Source: CAD feature listing. Evaluate the final solid. Frame: model axes, mm. A direction names the side the tool comes from. Coordinates: 2 decimals unless noted, no trailing zeros. Order: outer loops, then holes, each group sorted by start corner. A loop starts at its lowest first (then second) coordinate and runs counter-clockwise, first axis right, second up.
Item 1: Ray query, line 1 (Y direction, x = 28, z = 20); line 2 (Y direction, x = 8, z = -8.5); line 3 (X direction, y = 14.5, z = 4). Return the intervals inside material, ascending.
Item 2: Contact query for flat-ended pins moving along their axis: P1, Ø5, axis at x = -14, y = 18.5, coming from the -Z side; P2, Ø12, axis at y = 11, z = 6.5, coming from the -X side; P3, Ø10, axis at x = 6, z = 3.5, coming from the +Y side; P4, Ø8, axis at x = -18, z = -24, coming from the -Y side. Output: stop coordinate, or through.
Item 3: Section C-C on y = 10. Return the cut outline in (x, z).
Item 4: Section D-D on x = 25.4. Return the cut outline in (y, z).
Item 5: Reachability of faces 1 (the flat face through (0, 12.7, 2)), 2 (the flat face through (0, -25.4, 0)) from +Z, -Z, +X, -X, +Y, -Y: full face, straight path, thin tool, end or side. Return the list, or none.
Item 6: Section A-A on x = 0. Return the cut outline in (y, z).
Item 7: Section B-B on z = 0. Return the cut outline in (x, y).
Item 8: Mould query, pull axis Z, two halves, no side actions, for faces 3 (the cylindrical face through (3.86, -12.52, -5.04)), 4 (the flat face through (0, 6, 14.665)), 5 (the flat face through (-12.61, 6.26, -7.49)), 6 (the flat face through (8, 0, 0)). Classes: released by +Z, released by -Z, zero draft, split by the parting line, or undercut.
from build123d import *

# Parameters (mm, degrees)
BOSS_EXTRUDE1_DEPTH = 12.7
SKETCH2_R           = 12.7
BOSS_EXTRUDE2_DEPTH = 12.7
SKETCH3_R           = 6.35
BOSS_EXTRUDE3_DEPTH = 25.4


with BuildPart() as part:
    # Sketch1 → Boss-Extrude1 (new body)
    with BuildSketch(Plane(origin=(0, 0, 0), x_dir=(1, 0, 0), z_dir=(0, 1, 0))):
        with BuildLine():
            Line((-6.35, 18.330871047), (-19.05, -3.666174209))
            ThreePointArc((-19.05, -3.666174209), (-36.398522628, -21.014696837), (-12.7, -14.664696837))
            Line((-12.7, -14.664696837), (12.7, -14.664696837))
            ThreePointArc((12.7, -14.664696837), (36.398522628, -21.014696837), (19.05, -3.666174209))
            Line((19.05, -3.666174209), (6.35, 18.330871047))
            ThreePointArc((6.35, 18.330871047), (0, 42.029393675), (-6.35, 18.330871047))
        make_face()
    extrude(amount=BOSS_EXTRUDE1_DEPTH)

    # Sketch2 → Boss-Extrude2 (add)
    with BuildSketch(Plane(origin=(0, 12.7, 0), x_dir=(1, 0, 0), z_dir=(0, 1, 0))):
        with Locations(Location((-25.4, -14.664696837, 0), (0, 0, 60))):
            Circle(SKETCH2_R)
        with Locations(Location((25.4, -14.664696837, 0), (0, 0, 120))):
            Circle(SKETCH2_R)
        with Locations(Location((0, 29.329393675, 0), (0, 0, 240))):
            Circle(SKETCH2_R)
    extrude(amount=BOSS_EXTRUDE2_DEPTH)

    # Sketch3 → Boss-Extrude3 (add)
    with BuildSketch(Plane(origin=(0, 0, 0), x_dir=(-1, 0, 0), z_dir=(0, -1, 0))):
        with Locations(Location((0, 0, 0), (0, 0, 270))):
            Circle(SKETCH3_R)
    extrude(amount=BOSS_EXTRUDE3_DEPTH)


solid = part.part
Answer list:
1. line 1: y = 0 to 25.4
1. line 2: y = 0 to 12.7
1. line 3: x = -32.3 to -18.5, 18.5 to 32.3
2. P1: stops at z = -34.72
2. P2: stops at x = -37.91
2. P3: stops at y = 12.7
2. P4: passes through
3. outline: (-19.05, 3.67) - (-6.35, -18.33) arc R12.7 ccw (long way) to (6.35, -18.33) - (19.05, 3.67) arc R12.7 ccw (long way) to (12.7, 14.66) - (-12.7, 14.66) arc R12.7 ccw (long way) to start
4. outline: (0, 1.96) - (25.4, 1.96) - (25.4, 27.36) - (0, 27.36) - close
5. face 1: +Y
5. face 2: +Z, -Z, +X, -X, -Y
6. outline: (-25.4, -6.35) - (0, -6.35) - (0, -42.03) - (25.4, -42.03) - (25.4, -16.63) - (12.7, -16.63) - (12.7, 14.66) - (0, 14.66) - (0, 6.35) - (-25.4, 6.35) - close
7. outline: (-16.93, 0) - (-6.35, 0) - (-6.35, -25.4) - (6.35, -25.4) - (6.35, 0) - (16.93, 0) - (16.93, 12.7) - (-16.93, 12.7) - close
8. face 3: split by the parting line
8. face 4: released by +Z
8. face 5: undercut
8. face 6: zero draft
